Can you work these out from the drawing? Everything is in mm from the part's minimum corner. A direction names the side the tool comes from. Round coordinates to 2 decimals unless told otherwise and drop trailing zeros. Order: outer loops, then holes, each group sorted by start corner. A loop starts at its lowest first (then second) coordinate and runs counter-clockwise, first axis right, second up. Notation, with made-up numbers: M -5,44 L 36,44 A8 ccw 36,59 Z; hole C 79,-32 d2. An arc over 180 degrees is marked long. Use one line per item in the form item = value. Start each with the question number.
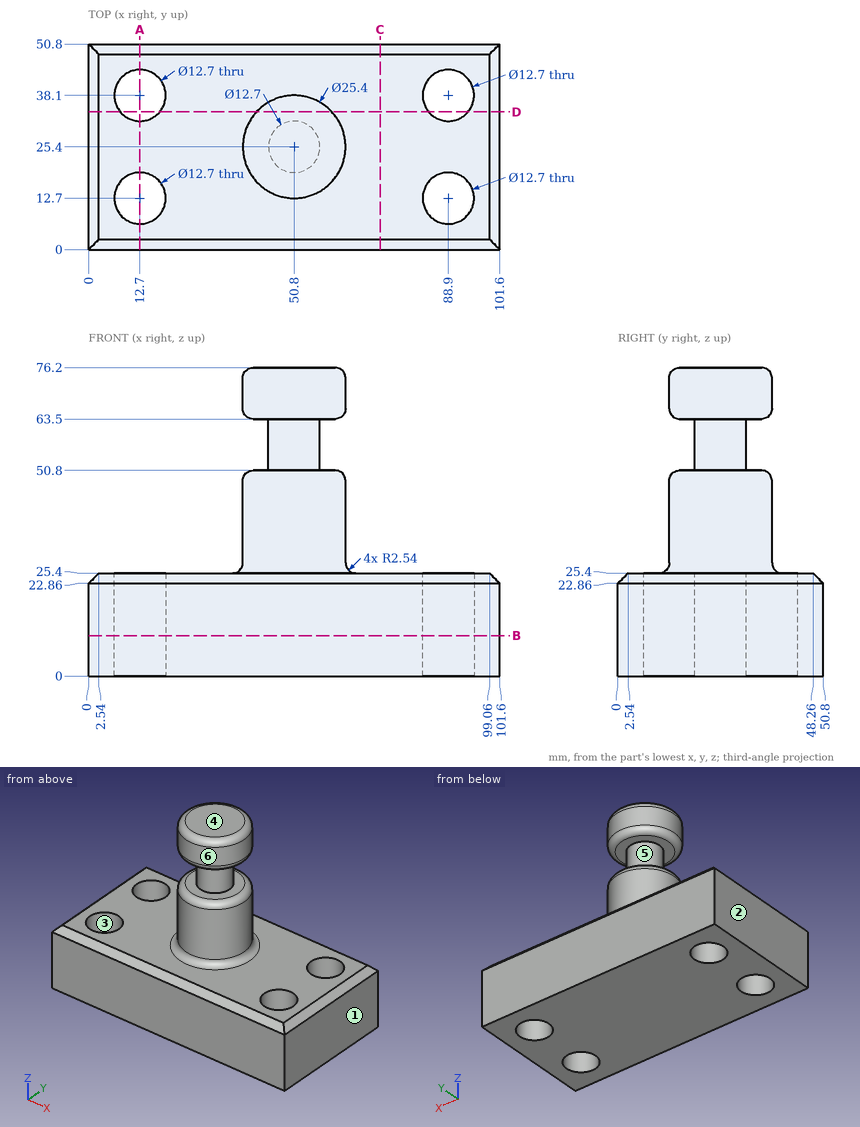
1) If we mould it in two halves opening along X, with no side actions, what happens to the marked faces 1, 2 and 3? For each: +X half, -X half, draft (parallel to the pull), parting line (faces both ways), or undercut.
2) Will these pins go through, and if not, where does the flat tip stop? pin 1 Ø8 at (x, y) = (43, 10) entering from +Z; pin 2 Ø16.5 at (x, y) = (12.7, 12.7) entering from +Z; pin 3 Ø5 at (x, y) = (25, 21.5) entering from -Z; pin 4 Ø12 at (y, z) = (31, 49.5) entering from +X.
3) If I drill on line 1 (X direction, y = 38, z = 15); line 2 (Y direction, x = 12.7, z = 17); line 3 (Z direction, x = 40.5, y = 26), over which ranges is the centre line in solid material (lowest first)?
4) If we section it at B-B on z = 10: Write out the boundary of the cut face in (x, y).
5) If we section it at D-D on y = 34: Give the number of separate pieces and of enclosed holes in the cut face, then the cut area to 3 significant figures.
6) If we section it at A-A on x = 12.7: Write out the boundary of the cut face in (y, z), then the cut area to 3 significant figures.
7) If we section it at C-C on x = 72: Write out the boundary of the cut face in (y, z).
8) On a 3-axis mill with a long thin cutter (end or side, diameter ignored), from which of +Z, -Z, +X, -X, +Y, -Y can I reach the whole of each face in a straight line? I mean the marked faces 4, 5 and 6. Say none if no direction works.
Completed:
q1.face_1 = +X half
q1.face_2 = -X half
q1.face_3 = undercut
q2.pin_1 = 26.35
q2.pin_2 = 25.4
q2.pin_3 = 0
q2.pin_4 = 63.5
q3.line_1 = 0 to 6.35, 19.05 to 82.55, 95.25 to 101.6
q3.line_2 = 0 to 6.35, 19.05 to 31.75, 44.45 to 50.8
q3.line_3 = 0 to 50.8, 63.5 to 76.2
q4.outline = M 0,0 L 101.6,0 L 101.6,50.8 L 0,50.8 Z; hole C 12.7,12.7 d12.7; hole C 12.7,38.1 d12.7; hole C 88.9,12.7 d12.7; hole C 88.9,38.1 d12.7
q5.separate_pieces = 4
q5.enclosed_holes = 0
q5.area = 2,790 mm²
q6.outline = M 0,0 L 6.35,0 L 6.35,25.4 L 2.54,25.4 L 0,22.86 Z; M 19.05,0 L 31.75,0 L 31.75,25.4 L 19.05,25.4 Z; M 44.45,0 L 50.8,0 L 50.8,22.86 L 48.26,25.4 L 44.45,25.4 Z
q6.area = 639 mm²
q7.outline = M 0,0 L 50.8,0 L 50.8,22.86 L 48.26,25.4 L 2.54,25.4 L 0,22.86 Z
q8.face_4 = +Z, +X, -X, +Y, -Y
q8.face_5 = none
q8.face_6 = +Z
